Model file for the job. Use its own axes, mm. A direction names the side the tool comes from. Coordinates: 2 decimals unless noted, no trailing zeros. Order: outer loops, then holes, each group sorted by start corner. A loop starts at its lowest first (then second) coordinate and runs counter-clockwise, first axis right, second up. Notation, with made-up numbers: (73, 72) -> (115, 72) arc R16 ccw to (115, 79) -> close; hole circle Ø3 at (-34.5, 86.25). An arc over 180 degrees is marked (long way). Return JSON: item names as keys, results as strings. Group by question number.
1) Which spindle directions (+Z, -Z, +X, -X, +Y, -Y) get a long thin tool onto all of the face, cutting with end or side? Do faces 1 (the flat face through (222.25, 17, 5)), 2 (the cylindrical face through (-157.86, 8.02, 9.45)), 3 (the flat face through (-69.85, 12, 0)), 4 (the flat face through (-1, 13, 47.117)), 5 (the flat face through (-90, 3.683, 42)). Say none if no direction does.
2) Cut at C-C (x = -143.5). Write the cut outline in (y, z).
3) Probe line 1 (X direction, y = 24.75, z = -5.5); line 2 (Z direction, x = -51, y = 9) (3 decimals); line 3 (X direction, y = 20, z = 15.5). List the from-to ranges inside material, lowest first.
4) Cut at B-B (x = 30). Write the cut outline in (y, z) (1 decimal).
5) Flat gauge pins, fed straight in: pin 1 (7 mm diameter, centred on x = 72, z = -26.5, fed in from +Y); pin 2 (5 mm diameter, centred on x = 74.5, z = 26.5, fed in from +Y); pin 3 (1.1 mm diameter, centred on y = 16.5, z = 16.5, fed in from -X); pin 4 (5 mm diameter, centred on y = 13, z = 23, fed in from +X). Where does each tip first touch, or does it go through?
from build123d import *

# Parameters (mm, degrees)
SKETCH2_W                                = 190.5
SKETCH2_H                                = 94.234
BOSS_EXTRUDE1_DEPTH                      = 25.4
SKETCH3_W                                = 152.4
SKETCH3_H                                = 60.96
CUT_EXTRUDE1_DEPTH                       = 7.7216
FILLET1_R                                = 2.286
CUT_EXTRUDE2_DEPTH                       = 1.9939
CUT_EXTRUDE3_DEPTH                       = 21.717
MIRROR1_AT_THE_SECOND_PLANE_COPY_1_DEPTH = 21.717
CUT_EXTRUDE6_DEPTH                       = 11.22531918
SKETCH10_R                               = 9.906
SKETCH10_R_2                             = 7.62
BOSS_EXTRUDE2_DEPTH                      = 127
CUT_EXTRUDE9_START                       = -25.4
SKETCH16_R                               = 7.62
CUT_EXTRUDE9_DEPTH                       = 25.4
BOSS_EXTRUDE3_REACH                      = 235.825


with BuildPart() as part:
    # Sketch2 → Boss-Extrude1 (new body)
    with BuildSketch(Plane(origin=(0, 0, 0), x_dir=(1, 0, 0), z_dir=(0, 1, 0))):
        Rectangle(SKETCH2_W, SKETCH2_H)
    extrude(amount=BOSS_EXTRUDE1_DEPTH)

    # Sketch3 → Cut-Extrude1 (cut)
    with BuildSketch(Plane(origin=(0, 25.4, 0), x_dir=(1, 0, 0), z_dir=(0, 1, 0))):
        Rectangle(SKETCH3_W, SKETCH3_H)
    extrude(amount=-CUT_EXTRUDE1_DEPTH, mode=Mode.SUBTRACT)

    # Fillet1
    fillet1_edges = [part.edges().sort_by_distance(p)[0] for p in [
        (76.2, 21.5392, -30.48),
        (76.2, 21.5392, 30.48),
        (-76.2, 21.5392, 30.48),
        (-76.2, 21.5392, -30.48),
    ]]
    fillet(fillet1_edges, radius=FILLET1_R)

    # Sketch5 → Cut-Extrude2 (cut)
    with BuildSketch(Plane(origin=(0, 25.4, 0), x_dir=(1, 0, 0), z_dir=(0, 1, 0))):
        with BuildLine():
            Line((-73.914, -35.3441), (73.914, -35.3441))
            ThreePointArc((73.914, -35.3441), (78.969884196, -33.249884196), (81.0641, -28.194))
            Line((81.0641, -28.194), (81.0641, 28.194))
            ThreePointArc((81.0641, 28.194), (78.969884196, 33.249884196), (73.914, 35.3441))
            Line((73.914, 35.3441), (-73.914, 35.3441))
            ThreePointArc((-73.914, 35.3441), (-78.969884196, 33.249884196), (-81.0641, 28.194))
            Line((-81.0641, 28.194), (-81.0641, -28.194))
            ThreePointArc((-81.0641, -28.194), (-78.969884196, -33.249884196), (-73.914, -35.3441))
        make_face()
        with BuildLine():
            Line((-73.914, -31.496), (73.914, -31.496))
            ThreePointArc((73.914, -31.496), (76.248866591, -30.528866591), (77.216, -28.194))
            Line((77.216, -28.194), (77.216, 28.194))
            ThreePointArc((77.216, 28.194), (76.248866591, 30.528866591), (73.914, 31.496))
            Line((73.914, 31.496), (-73.914, 31.496))
            ThreePointArc((-73.914, 31.496), (-76.248866591, 30.528866591), (-77.216, 28.194))
            Line((-77.216, 28.194), (-77.216, -28.194))
            ThreePointArc((-77.216, -28.194), (-76.248866591, -30.528866591), (-73.914, -31.496))
        make_face(mode=Mode.SUBTRACT)
    extrude(amount=-CUT_EXTRUDE2_DEPTH, mode=Mode.SUBTRACT)

    # Sketch6 → Cut-Extrude3 (cut)
    with BuildSketch(Plane(origin=(0, 25.4, 0), x_dir=(1, 0, 0), z_dir=(0, 1, 0))):
        with BuildLine():
            Line((-84.328, 47.117), (-84.328, 42.545))
            ThreePointArc((-84.328, 42.545), (-86.187871939, 38.054871939), (-90.678, 36.195))
            Line((-90.678, 36.195), (-95.25, 36.195))
            Line((-95.25, 36.195), (-95.25, 47.117))
            Line((-95.25, 47.117), (-84.328, 47.117))
        make_face()
    cut_extrude3 = extrude(amount=-CUT_EXTRUDE3_DEPTH, mode=Mode.SUBTRACT)

    # Mirror1: Cut-Extrude3 across plane
    add(cut_extrude3.mirror(Plane(origin=(0, 0, 0), x_dir=(0, 0, 1), z_dir=(1, 0, 0))), mode=Mode.SUBTRACT)

    # Mirror1 at the second plane: Cut-Extrude3 across plane
    add(cut_extrude3.mirror(Plane.XY), mode=Mode.SUBTRACT)

    # Mirror1 at the second plane copy 1 sketc → Mirror1 at the second plane copy 1 (cut)
    with BuildSketch(Plane(origin=(0, 25.4, 0), x_dir=(-1, 0, 0), z_dir=(0, 1, 0))):
        with BuildLine():
            Line((-84.328, 47.117), (-84.328, 42.545))
            ThreePointArc((-84.328, 42.545), (-86.187871939, 38.054871939), (-90.678, 36.195))
            Line((-90.678, 36.195), (-95.25, 36.195))
            Line((-95.25, 36.195), (-95.25, 47.117))
            Line((-95.25, 47.117), (-84.328, 47.117))
        make_face()
    extrude(amount=-MIRROR1_AT_THE_SECOND_PLANE_COPY_1_DEPTH, mode=Mode.SUBTRACT)

    # Sketch13 → Cut-Extrude6 (cut)
    with BuildSketch(Plane(origin=(0, 17.6784, 0), x_dir=(1, 0, 0), z_dir=(0, 1, 0))):
        with BuildLine():
            Line((-63.000000018, 24.13), (63.5, 24.13))
            ThreePointArc((63.5, 24.13), (67.990128061, 22.270128061), (69.85, 17.78))
            Line((69.85, 17.78), (69.85, -17.78))
            ThreePointArc((69.85, -17.78), (67.990128061, -22.270128061), (63.5, -24.13))
            Line((63.5, -24.13), (-63.000000018, -24.13))
            ThreePointArc((-63.000000018, -24.13), (-66.175000018, -27.305), (-63.000000018, -30.48))
            Line((-63.000000018, -30.48), (69.85, -30.48))
            ThreePointArc((69.85, -30.48), (74.340128061, -28.620128061), (76.2, -24.13))
            Line((76.2, -24.13), (76.2, 24.13))
            ThreePointArc((76.2, 24.13), (74.340128061, 28.620128061), (69.85, 30.48))
            Line((69.85, 30.48), (-63.000000018, 30.48))
            ThreePointArc((-63.000000018, 30.48), (-66.175000018, 27.305), (-63.000000018, 24.13))
        make_face()
        with BuildLine():
            Line((-66.580399175, 24.13), (-63.000000018, 24.13))
            ThreePointArc((-63.000000018, 24.13), (-66.175000018, 27.305), (-63.000000018, 30.48))
            Line((-63.000000018, 30.48), (-66.580399175, 30.48))
            Line((-66.580399175, 30.48), (-66.580399175, 24.13))
        make_face()
        with BuildLine():
            Line((-76.2, 14.605), (-76.2, -14.605))
            ThreePointArc((-76.2, -14.605), (-74.340128061, -19.095128061), (-69.85, -20.955))
            Line((-69.85, -20.955), (63.000000018, -20.955))
            ThreePointArc((63.000000018, -20.955), (66.175000018, -17.78), (63.000000018, -14.605))
            Line((63.000000018, -14.605), (-63.5, -14.605))
            ThreePointArc((-63.5, -14.605), (-67.990128061, -12.745128061), (-69.85, -8.255))
            Line((-69.85, -8.255), (-69.85, 8.255))
            ThreePointArc((-69.85, 8.255), (-67.990128061, 12.745128061), (-63.5, 14.605))
            Line((-63.5, 14.605), (63.000000018, 14.605))
            ThreePointArc((63.000000018, 14.605), (66.175000018, 17.78), (63.000000018, 20.955))
            Line((63.000000018, 20.955), (-69.85, 20.955))
            ThreePointArc((-69.85, 20.955), (-74.340128061, 19.095128061), (-76.2, 14.605))
        make_face()
        with BuildLine():
            Line((63.000000018, 20.955), (66.84830001, 20.955))
            Line((66.84830001, 20.955), (66.84830001, 14.605))
            Line((66.84830001, 14.605), (63.000000018, 14.605))
            ThreePointArc((63.000000018, 14.605), (66.175000018, 17.78), (63.000000018, 20.955))
        make_face()
        with BuildLine():
            ThreePointArc((63.000000018, -20.955), (66.175000018, -17.78), (63.000000018, -14.605))
            Line((63.000000018, -14.605), (66.84830001, -14.605))
            Line((66.84830001, -14.605), (66.84830001, -20.955))
            Line((66.84830001, -20.955), (63.000000018, -20.955))
        make_face()
        with BuildLine():
            ThreePointArc((-63.000000018, -30.48), (-66.175000018, -27.305), (-63.000000018, -24.13))
            Line((-63.000000018, -24.13), (-66.580399175, -24.13))
            Line((-66.580399175, -24.13), (-66.580399175, -30.48))
            Line((-66.580399175, -30.48), (-63.000000018, -30.48))
        make_face()
    extrude(amount=-CUT_EXTRUDE6_DEPTH, mode=Mode.SUBTRACT)

    # Sketch10 → Boss-Extrude2 (add)
    with BuildSketch(Plane(origin=(95.25, 0, 0), x_dir=(0, 0, -1), z_dir=(1, 0, 0))):
        with Locations(Location((0, 10.996509823, 0), (0, 0, 180))):
            Circle(SKETCH10_R)
        with Locations((0, 10.996509823)):
            Circle(SKETCH10_R_2, mode=Mode.SUBTRACT)
    boss_extrude2 = extrude(amount=BOSS_EXTRUDE2_DEPTH)

    # Sketch16 → Cut-Extrude9 (cut)
    with BuildSketch(Plane(origin=(95.25, 0, 0), x_dir=(0, 0, -1), z_dir=(1, 0, 0)).offset(CUT_EXTRUDE9_START)):
        with Locations(Location((0, 10.996509823, 0), (0, 0, 216.601830643))):
            Circle(SKETCH16_R)
    cut_extrude9 = extrude(amount=CUT_EXTRUDE9_DEPTH, mode=Mode.SUBTRACT)

    # Mirror2: Boss-Extrude2, Cut-Extrude9 across plane
    add(boss_extrude2.mirror(Plane(origin=(0, 0, 0), x_dir=(0, 0, 1), z_dir=(1, 0, 0))))
    add(cut_extrude9.mirror(Plane(origin=(0, 0, 0), x_dir=(0, 0, 1), z_dir=(1, 0, 0))), mode=Mode.SUBTRACT)

    # Boss-Extrude3: up to this face of the body (flat: up to its plane)
    boss_extrude3_end = Plane(part.part.faces().sort_by_distance((-1.500849995, 12.06574041, 20.955))[0])
    # Sketch17 → Boss-Extrude3 (add, up to the picked face)
    with BuildSketch(Plane.XY.offset(-20.955), mode=Mode.PRIVATE) as boss_extrude3_sk1:
        Polygon((66.84830001, 6.45308082), (66.84830001, 15.43307302), (-63.5, 6.45308082), align=None)
    boss_extrude3_tool1 = split(extrude(boss_extrude3_sk1.sketch, amount=BOSS_EXTRUDE3_REACH, mode=Mode.PRIVATE), bisect_by=boss_extrude3_end, keep=Keep.BOTH, mode=Mode.PRIVATE)
    add(boss_extrude3_tool1.solids().sort_by(Axis((23.398867, 9.446412, -20.955), (0, 0, 1)))[0])


solid = part.part
Answers below:
{
 "1": {"face 1": "+Z, -Z, +X, +Y, -Y", "face 2": "-X", "face 3": "+Y", "face 4": "+Z, +X, -X, +Y, -Y", "face 5": "+Z, -X, +Y"},
 "2": {"outline": "circle Ø19.81 at (11, 0); hole circle Ø15.24 at (11, 0)"},
 "3": {"line 1": "x = -95.25 to -81.06, -77.22 to -76.2, 76.2 to 77.22, 81.06 to 95.25", "line 2": "z = -47.117 to -30.48, -24.13 to -20.955, -14.605 to 14.605, 20.955 to 24.13, 30.48 to 47.117", "line 3": "x = -95.25 to -76.2, 76.2 to 95.25"},
 "4": {"outline": "(0, -47.1) -> (25.4, -47.1) -> (25.4, -35.3) -> (23.4, -35.3) -> (23.4, -31.5) -> (25.4, -31.5) -> (25.4, -30.5) -> (6.5, -30.5) -> (6.5, -24.1) -> (17.7, -24.1) -> (17.7, -21) -> (12.9, -21) -> (12.9, -14.6) -> (17.7, -14.6) -> (17.7, 14.6) -> (12.9, 14.6) -> (12.9, 21) -> (17.7, 21) -> (17.7, 24.1) -> (6.5, 24.1) -> (6.5, 30.5) -> (25.4, 30.5) -> (25.4, 31.5) -> (23.4, 31.5) -> (23.4, 35.3) -> (25.4, 35.3) -> (25.4, 47.1) -> (0, 47.1) -> close"},
 "5": {"pin 1": "stops at y = 17.68", "pin 2": "stops at y = 25.4", "pin 3": "stops at x = -95.25", "pin 4": "stops at x = 95.25"}
}
